The model under review builds one solid part; all positions refer to its coordinate system, in mm. A direction names the side the tool comes from. Round coordinates to 2 decimals unless told otherwise and drop trailing zeros. Write each loop counter-clockwise with the first axis right and the second up, starting at its lowest first coordinate (ties: lowest second). Pieces come first, ordered by that corner, then holes. Notation, with made-up numbers: (86, -15) -> (101, -15) arc R34 ccw to (101, 24) -> close; hole circle Ø10 at (-10.5, 71). An arc over 180 degrees is marked (long way). Return JSON: item names as keys, results as strings. Group by question number.
1. Take a section at B-B, the plane z = -8.5. Write out the cut boundary in (x, y).
2. Take a section at C-C, the plane z = -17. Give the number of separate pieces and of enclosed holes in the cut face, then the cut area to 3 significant figures.
3. For line 1 along X through (y, z) = (13.75, 9); line 2 along Y through (x, z) = (-8, -17.5); line 3 along Y through (x, z) = (-25.5, -18), list the stretches that pass through material, from the lowest coordinate up. Write a range as from..to.
4. Tool access review of faces 1 (the conical face through (-25.292, 2.004, 11.716)), 2 (the flat face through (-24.5, 3, -5)), 3 (the flat face through (-25.514, 11.148, 12.778)), 4 (the flat face through (-26, 22, -7)), 5 (the flat face through (-1.607, 2.535, -17.381)): name each direction out of +Z, -Z, +X, -X, +Y, -Y from which nothing blocks a thin tool from reaching the whole face with its end or side.
5. Take a section at A-A, the plane y = 15.25. Write out the cut boundary in (x, z), then the cut area to 3 significant figures.
6. Take a section at D-D, the plane x = -8. Write out the cut boundary in (y, z), then the cut area to 3 significant figures.
7. Mouldability with a two-part tool opening along Y and no side actions: class faces 6 (the flat face through (-20, 3, -21.486)), 7 (the flat face through (-28, 11, -16.236)), 8 (the flat face through (30, 22, -7)) as pulls with the +Y half, pulls with the -Y half, needs draft (parallel to the pull), parting line crosses it, or undercut.
8. Clearance check with flat-ended pins moving along their axes: P1, Ø2.5, axis at x = 4.5, y = 3, coming from the +Z side; P2, Ø4, axis at y = 15, z = -13, coming from the +X side. State where each tip first meets the part, or that it passes through.
Autodesk Inventor part; units mm, degrees
ref_plane "YZ Plane" through (0, 0, 0) normal (1, 0, 0) x (0, 1, 0)
ref_plane "XZ Plane" through (0, 0, 0) normal (0, 1, 0) x (-1, 0, 0)
ref_plane "XY Plane" through (0, 0, 0) normal (0, 0, 1) x (1, 0, 0)
sketch "Boceto1" plane through (0, 0, 0) normal (0, 1, 0) x (-1, 0, 0)
  line L0 (29.505, -15) -> (44.5466, 0) construction
  line L1 (33.6552, -19.1617) -> (29.505, -15) construction
  line L2 (0, 0) -> (0, 6.3504) construction
  line L3 (0, 0) -> (0, -23.2363) construction
  line L4 (0, -14.2363) -> (24.5, -14.2363)
  line L5 (31.5, -23.2363) -> (31.5, 13.7637)
  line L6 (31.5, 13.7637) -> (24.5, 13.7637)
  line L7 (24.5, 13.7637) -> (24.5, -14.2363)
  line L8 (31.5, -23.2363) -> (0, -23.2363)
  line L9 (0, -14.2363) -> (-24.5, -14.2363)
  line L10 (-31.5, -23.2363) -> (-31.5, 13.7637)
  line L11 (-31.5, 13.7637) -> (-24.5, 13.7637)
  line L12 (-24.5, 13.7637) -> (-24.5, -14.2363)
  line L13 (-31.5, -23.2363) -> (0, -23.2363)
  dimension "d70" = 7
  dimension "d71" = 37
  dimension "d86" = 31.5
  dimension "d88" = 9
extrude "Extrusión1" add sketch "Boceto1" along normal blind 5
sketch "Boceto11" plane through (0, 5, 0) normal (0, 1, 0) x (1, 0, 0)
  line L0 (-31.5, -13.7637) -> (-24.5, -13.7637)
  line L1 (31.5, 23.2363) -> (-31.5, 23.2363)
  line L2 (-31.5, -13.7637) -> (-24.5, -13.7637)
  line L3 (-24.5, -13.7637) -> (-24.5, 23.2363)
  line L4 (-24.5, 23.2363) -> (-31.5, 23.2363)
  line L5 (-31.5, 23.2363) -> (-31.5, -13.7637)
  line L6 (0, 0) -> (0, -8.2135) construction
  line L7 (31.5, -13.7637) -> (24.5, -13.7637)
  line L8 (24.5, -13.7637) -> (24.5, 23.2363)
  line L9 (24.5, 23.2363) -> (31.5, 23.2363)
  line L10 (31.5, 23.2363) -> (31.5, -13.7637)
  point P0 (31.5, 23.2363)
  point P1 (24.5, 23.2363)
extrude "Extrusión7" add sketch "Boceto11" along normal blind 17.5
sketch "Boceto12" plane through (31.5, 0, 13.7637) normal (1, 0, 0) x (0, 0, -1)
  line L0 (7, 17.5) -> (30, 17.5)
  line L1 (30, 17.5) -> (30, 5)
  line L2 (30, 5) -> (7, 5)
  line L3 (7, 5) -> (7, 17.5)
  line L4 (37, 22.5) -> (0, 22.5)
  line L5 (18.5, 22.5) -> (18.5, 29.9213) construction
  line L6 (0, 0) -> (0, 22.5)
  line L7 (0, 11.25) -> (-3.0724, 11.25) construction
  point P0 (13.7637, 0)
  dimension "d74" = 12.5
  dimension "d75" = 23
extrude "Extrusión8" cut sketch "Boceto12" against normal through all
fillet "Empalme5" radius 4 4 edges at (-28, 0, 13.7637) (-28, 22.5, 13.7637) (28, 0, 13.7637) (28, 22.5, 13.7637)
chamfer "Chaflán3" distance 2 angle 45 20 edges at (31.5, 22.5, -6.7363) (31.5, 21.3284, 12.5921) (31.5, 11.25, 13.7637) (31.5, 1.1716, 12.5921) (31.5, 0, -6.7363) (-31.5, 22.5, -6.7363) (-31.5, 21.3284, 12.5921) (-31.5, 11.25, 13.7637) (-31.5, 1.1716, 12.5921) (-31.5, 0, -6.7363) (-24.5, 22.5, -6.7363) (-24.5, 21.3284, 12.5921) (-24.5, 11.25, 13.7637) (-24.5, 1.1716, 12.5921) (-24.5, 0, -2.2363) (24.5, 22.5, -6.7363) (24.5, 21.3284, 12.5921) (24.5, 11.25, 13.7637) (24.5, 1.1716, 12.5921) (24.5, 0, -2.2363)
sketch "Boceto13" plane through (0, 5, 0) normal (0, 1, 0) x (1, 0, 0)
  line L0 (0, 0) -> (0, -6.0566) construction
  line L1 (-2.4123, 15.9863) -> (-5.5877, 15.9863)
  line L2 (-5.5877, 15.9863) -> (-7.1754, 18.7363)
  line L3 (-7.1754, 18.7363) -> (-5.5877, 21.4863)
  line L4 (-5.5877, 21.4863) -> (-2.4123, 21.4863)
  line L5 (-2.4123, 21.4863) -> (-0.8246, 18.7363)
  line L6 (-0.8246, 18.7363) -> (-2.4123, 15.9863)
  line L7 (24.5, 23.2363) -> (-24.5, 23.2363)
  line L8 (-13.5877, 21.4863) -> (-10.4123, 21.4863)
  line L9 (-15.1754, 18.7363) -> (-13.5877, 21.4863)
  line L10 (-13.5877, 15.9863) -> (-15.1754, 18.7363)
  line L11 (-10.4123, 15.9863) -> (-13.5877, 15.9863)
  line L12 (-8.8246, 18.7363) -> (-10.4123, 15.9863)
  line L13 (-10.4123, 21.4863) -> (-8.8246, 18.7363)
  line L14 (-21.5877, 21.4863) -> (-18.4123, 21.4863)
  line L15 (-23.1754, 18.7363) -> (-21.5877, 21.4863)
  line L16 (-21.5877, 15.9863) -> (-23.1754, 18.7363)
  line L17 (-18.4123, 15.9863) -> (-21.5877, 15.9863)
  line L18 (-16.8246, 18.7363) -> (-18.4123, 15.9863)
  line L19 (-18.4123, 21.4863) -> (-16.8246, 18.7363)
  line L20 (2.4123, 15.9863) -> (5.5877, 15.9863)
  line L21 (5.5877, 15.9863) -> (7.1754, 18.7363)
  line L22 (7.1754, 18.7363) -> (5.5877, 21.4863)
  line L23 (5.5877, 21.4863) -> (2.4123, 21.4863)
  line L24 (2.4123, 21.4863) -> (0.8246, 18.7363)
  line L25 (0.8246, 18.7363) -> (2.4123, 15.9863)
  line L26 (13.5877, 21.4863) -> (10.4123, 21.4863)
  line L27 (15.1754, 18.7363) -> (13.5877, 21.4863)
  line L28 (13.5877, 15.9863) -> (15.1754, 18.7363)
  line L29 (10.4123, 15.9863) -> (13.5877, 15.9863)
  line L30 (8.8246, 18.7363) -> (10.4123, 15.9863)
  line L31 (10.4123, 21.4863) -> (8.8246, 18.7363)
  line L32 (21.5877, 21.4863) -> (18.4123, 21.4863)
  line L33 (23.1754, 18.7363) -> (21.5877, 21.4863)
  line L34 (21.5877, 15.9863) -> (23.1754, 18.7363)
  line L35 (18.4123, 15.9863) -> (21.5877, 15.9863)
  line L36 (16.8246, 18.7363) -> (18.4123, 15.9863)
  line L37 (18.4123, 21.4863) -> (16.8246, 18.7363)
  point P0 (-4, 18.7363)
  dimension "d87" = 5.5
  dimension "d89" = 4.5
  dimension "d90" = 4
  dimension "d93" = 8
extrude "Extrusión9" cut sketch "Boceto13" against normal up to surface (5 mm away)
properties part number "Chassis_atras_V4"
Output:
{
 "1": {"outline": "(-31.5, 2) -> (-29.5, 0) -> (-26.5, 0) -> (-24.5, 2) -> (-24.5, 5) -> (-31.5, 5) -> close; (-31.5, 17.5) -> (-24.5, 17.5) -> (-24.5, 20.5) -> (-26.5, 22.5) -> (-29.5, 22.5) -> (-31.5, 20.5) -> close; (24.5, 2) -> (26.5, 0) -> (29.5, 0) -> (31.5, 2) -> (31.5, 5) -> (24.5, 5) -> close; (24.5, 17.5) -> (31.5, 17.5) -> (31.5, 20.5) -> (29.5, 22.5) -> (26.5, 22.5) -> (24.5, 20.5) -> close"},
 "2": {"separate pieces": "7", "enclosed holes": "0", "area": "418 mm^2"},
 "3": {"line 1": "x = -31.5..-24.5, 24.5..31.5", "line 2": "y = 0..5", "line 3": "y = 0..21.5"},
 "4": {"face 1": "+Z, -Y", "face 2": "+Z, +Y", "face 3": "+Z, +Y, -Y", "face 4": "+Z, -Z, +Y", "face 5": "+Y, -Y"},
 "5": {"outline": "(-31.5, -23.24) -> (-24.5, -23.24) -> (-24.5, -16.24) -> (-31.5, -16.24) -> close; (-31.5, 6.76) -> (-24.5, 6.76) -> (-24.5, 11.76) -> (-26.5, 13.76) -> (-29.5, 13.76) -> (-31.5, 11.76) -> close; (24.5, -23.24) -> (31.5, -23.24) -> (31.5, -16.24) -> (24.5, -16.24) -> close; (24.5, 6.76) -> (31.5, 6.76) -> (31.5, 11.76) -> (29.5, 13.76) -> (26.5, 13.76) -> (24.5, 11.76) -> close", "area": "188 mm^2"},
 "6": {"outline": "(0, -23.24) -> (5, -23.24) -> (5, -14.24) -> (0, -14.24) -> close", "area": "45.0 mm^2"},
 "7": {"face 6": "needs draft", "face 7": "undercut", "face 8": "pulls with the +Y half"},
 "8": {"P1": "stops at z = -14.24", "P2": "passes through"}
}
